The model under review builds one solid part; all positions refer to its coordinate system, in mm. A direction names the side the tool comes from. Round coordinates to 2 decimals unless told otherwise and drop trailing zeros. Order: outer loops, then holes, each group sorted by start corner. A loop starts at its lowest first (then second) coordinate and runs counter-clockwise, first axis right, second up.
1) Consider section D-D (y = -3.25). Give the boundary of the cut face in (x, z), then the cut area to 3 significant figures.
2) Consider section B-B (y = 0). Give the boundary of the cut face in (x, z) (3 decimals), then the cut area to 3 significant figures.
3) Consider section A-A (x = -2). Give the boundary of the cut face in (y, z), then the cut area to 3 significant figures.
4) Clearance check with flat-ended pins moving along their axes: P1, Ø3, axis at x = -2, y = 2, coming from the +Z side; P2, Ø1.5, axis at x = 4, z = 17, coming from the -Y side; P3, Ø3, axis at y = -2.5, z = 8, coming from the -X side. State where each tip first meets the part, or that it passes through.
5) Consider section C-C (z = 28). Give the boundary of the cut face in (x, y) (3 decimals), then the cut area to 3 significant figures.
6) To check wall thickness, follow L1, parallel to Y at x = 0, z = 30.25 (3 decimals); L2, parallel to Y at x = 0, z = 16 (3 decimals); L3, parallel to Z at x = 4, y = -1.5. State the ranges of each line that lie inside material, in increasing order.
7) Mouldability with a two-part tool opening along Y and no side actions: class faces 3 (the face through (-0.1, -3.2, 27)), 4 (the face through (-1.08, 4.88, -1.73)), 5 (the face through (-5, -2, 0)) as pulls with the +Y half, pulls with the -Y half, needs draft (parallel to the pull), parting line crosses it, or undercut.
8) Machinability: for faces 1 (the face through (-2.9, -0.1, 12)), 2 (the face through (-0.635, 4.834, 30.549)), which of the approach directions +Z, -Z, +X, -X, +Y, -Y give a long, thin tool a straight path to every point of the face, cutting with its end or side? Answer none if there is none.
from build123d import *

# Parameters (mm, degrees)
F0_R     = 6.875
F0_R_2   = 2.9
F1_DEPTH = 34
F2_R     = 5
F2_R_2   = 2.9
F3_DEPTH = 3.5
F4_R     = 4.875
F5_DEPTH = 7


with BuildPart() as f1:
    # F0 (on Top) → F1 (new body)
    with BuildSketch(Plane.XY):
        Circle(F0_R)
        Circle(F0_R_2, mode=Mode.SUBTRACT)
    extrude(amount=F1_DEPTH)

    # F2 (on face) → F3 (join)
    with BuildSketch(Plane(origin=(0, 0, 0), x_dir=(1, 0, 0), z_dir=(0, 0, -1))):
        Circle(F2_R)
        Circle(F2_R_2, mode=Mode.SUBTRACT)
    extrude(amount=F3_DEPTH)

    # F4 (on face) → F5 (cut)
    with BuildSketch(Plane.XY.offset(34)):
        Circle(F4_R)
    extrude(amount=-F5_DEPTH, mode=Mode.SUBTRACT)


solid = f1.part
Answer below:
1. outline: (-6.06, 0) - (-3.8, 0) - (-3.8, -3.5) - (3.8, -3.5) - (3.8, 0) - (6.06, 0) - (6.06, 34) - (3.63, 34) - (3.63, 27) - (-3.63, 27) - (-3.63, 34) - (-6.06, 34) - close
1. area: 388 mm2
2. outline: (-6.875, 0) - (-5, 0) - (-5, -3.5) - (-2.9, -3.5) - (-2.9, 27) - (-4.875, 27) - (-4.875, 34) - (-6.875, 34) - close; (2.9, -3.5) - (5, -3.5) - (5, 0) - (6.875, 0) - (6.875, 34) - (4.875, 34) - (4.875, 27) - (2.9, 27) - close
2. area: 257 mm2
3. outline: (-6.58, 0) - (-4.58, 0) - (-4.58, -3.5) - (-2.1, -3.5) - (-2.1, 27) - (-4.45, 27) - (-4.45, 34) - (-6.58, 34) - close; (2.1, -3.5) - (4.58, -3.5) - (4.58, 0) - (6.58, 0) - (6.58, 34) - (4.45, 34) - (4.45, 27) - (2.1, 27) - close
3. area: 289 mm2
4. P1: stops at z = 27
4. P2: stops at y = -6.06
4. P3: stops at x = -6.8
5. outline: circle Ø13.75 at (0, 0); hole circle Ø9.75 at (0, 0)
5. area: 73.8 mm2
6. L1: y = -6.875 to -4.875, 4.875 to 6.875
6. L2: y = -6.875 to -2.9, 2.9 to 6.875
6. L3: z = -3.5 to 27
7. face 3: undercut
7. face 4: parting line crosses it
7. face 5: needs draft
8. face 1: +Z, -Z
8. face 2: +Z
